The listing builds one solid part. Answer for the finished solid, in the listing's coordinates (mm). A direction names the side the tool comes from. Coordinates: 2 decimals unless noted, no trailing zeros. Order: outer loops, then holes, each group sorted by start corner. A loop starts at its lowest first (then second) coordinate and runs counter-clockwise, first axis right, second up. Notation, with made-up numbers: M 82.5,77 L 112.5,77 A23 ccw 112.5,91 Z; hole C 50,52.5 d3. An arc over 180 degrees is marked long. One line per item, written item: value. Start each with the question number.
Q1. The part is cut by section C-C on z = 12.6. Give the vertices of the cut face in (x, y), then the cut area to 3 significant figures.
Q2. Each of these flat-tipped pins is pushed along its axis until it touches: pin 1 Ø5 at (x, y) = (-13, 33) entering from -Z; pin 2 Ø12.5 at (y, z) = (13.5, 10) entering from -X; pin 3 Ø0.9 at (y, z) = (45.5, 35.5) entering from -X. Where does it stop, or does it pass through?
Q3. For faces 5 (the flat face through (-23.42, 54.41, 32.84)), 6 (the flat face through (1, 33, 0)), 7 (the flat face through (-29, 45, 35)), 8 (the flat face through (-19.5, 52, 29)), determine the directions among +Z, -Z, +X, -X, +Y, -Y from which every point of the face is accessible in a straight line to the end or side of a thin tool.
Q4. The part is cut by section B-B on y = 3.5. Give the vertices of the cut face in (x, z), then the cut area to 3 significant figures.
Q5. Determine the mould class of faces 1 (the flat face through (-28.65, 54.59, 33.86)), 2 (the flat face through (-9, 11, 12)), 3 (the cylindrical face through (-51.59, 52.94, 13.09)), 4 (the cylindrical face through (-57.526, 52.944, -2.419)) for opening direction X: pulls with the +X half, pulls with the -X half, needs draft (parallel to the pull), parting line crosses it, or undercut.
Q6. Straight lines are drawn through the part: line 1 along Y through (x, z) = (-44, 34); line 2 along Z through (x, y) = (3, 3); line 3 along Z through (x, y) = (-17, 18). For each, find the intervals that lie inside material, in ascending order. Write a range as [from, to].
Q7. The part is cut by section D-D on x = 4. Give the vertices of the cut face in (y, z).
Q8. The part is cut by section A-A on z = 28.1. Give the vertices of the cut face in (x, y).
```python
from build123d import *

# Parameters (mm, degrees)
BOSS_EXTRUDE1_DEPTH = 25.2
SKETCH2_R           = 1.6
BOSS_EXTRUDE2_DEPTH = 6
SKETCH3_W           = 19
SKETCH3_H           = 1
CUT_EXTRUDE1_DEPTH  = 38.2
CHAMFER2_SIZE       = 1.55
SKETCH4_R           = 11.1
CUT_EXTRUDE2_DEPTH  = 86.626222619
CHAMFER3_SIZE       = 1.55
CHAMFER4_SIZE       = 1
SKETCH5_R           = 1.6
CUT_EXTRUDE3_DEPTH  = 96.48869043
SKETCH6_W           = 20
SKETCH6_H           = 15
BOSS_EXTRUDE3_DEPTH = 3
SKETCH7_R           = 0.9
CUT_EXTRUDE4_DEPTH  = 95.097236941
CHAMFER7_SIZE       = 1.55
CHAMFER8_SIZE       = 1.55
SKETCH8_W           = 0.2
SKETCH8_H           = 55.2
CUT_EXTRUDE5_DEPTH  = 90.209024207
CHAMFER9_SIZE       = 1.6


with BuildPart() as part:
    # Sketch1 → Boss-Extrude1 (new body)
    with BuildSketch(Plane.XY):
        Polygon((0, 0), (0, 11), (-19, 11), (-19, 49.2), (8.8, 49.2), (8.8, 0), align=None)
    extrude(amount=BOSS_EXTRUDE1_DEPTH)

    # Sketch2 → Boss-Extrude2 (add)
    with BuildSketch(Plane(origin=(0, 49.2, 0), x_dir=(1, 0, 0), z_dir=(0, 1, 0))):
        Polygon((-61.5, 8.4), (-19.5, 8.4), (-19.5, 0), (8.8, 0), (8.8, -25.2), (-19.5, -25.2), (-19.5, -33.6), (-61.5, -33.6), align=None)
        with Locations(Location((-56, 2.9, 0), (0, 0, 180))):
            Circle(SKETCH2_R, mode=Mode.SUBTRACT)
        with Locations((-56, -28.1)):
            Circle(SKETCH2_R, mode=Mode.SUBTRACT)
        with Locations(Location((-25, -28.1, 0), (0, 0, 180))):
            Circle(SKETCH2_R, mode=Mode.SUBTRACT)
        with Locations((-25, 2.9)):
            Circle(SKETCH2_R, mode=Mode.SUBTRACT)
    extrude(amount=BOSS_EXTRUDE2_DEPTH)

    # Sketch3 → Cut-Extrude1 (cut)
    with BuildSketch(Plane.XZ.offset(-11)):
        with Locations((-9.5, 24.7)):
            Rectangle(SKETCH3_W, SKETCH3_H)
        with Locations((-9.5, 0.5)):
            Rectangle(SKETCH3_W, SKETCH3_H)
    extrude(amount=-CUT_EXTRUDE1_DEPTH, mode=Mode.SUBTRACT)

    # Chamfer2
    chamfer2_edges = [part.edges().sort_by_distance(p)[0] for p in [
        (-54.4, 49.2, -2.9),
        (-57.6, 49.2, 28.1),
        (-23.4, 49.2, 28.1),
        (-26.6, 49.2, -2.9),
    ]]
    chamfer(chamfer2_edges, length=CHAMFER2_SIZE)

    # Sketch4 → Cut-Extrude2 (cut, through all)
    with BuildSketch(Plane.XZ.offset(-49.2)):
        with Locations((-40.5, 12.6)):
            Circle(SKETCH4_R)
    extrude(amount=-CUT_EXTRUDE2_DEPTH, mode=Mode.SUBTRACT)

    # Chamfer3
    chamfer3_edges = [part.edges().sort_by_distance(p)[0] for p in [
        (-61.5, 55.2, 12.6),
        (-19.5, 52.2, 0),
        (-19.5, 52.2, -8.4),
        (-61.5, 49.2, 12.6),
        (-61.5, 52.2, -8.4),
        (-61.5, 52.2, 33.6),
        (-19.5, 52.2, 33.6),
        (-19.5, 52.2, 25.2),
        (-19, 30.1, 24.2),
        (-19, 30.1, 1),
        (-51.6, 49.2, 12.6),
    ]]
    chamfer(chamfer3_edges, length=CHAMFER3_SIZE)

    # Chamfer4
    chamfer4_edges = [part.edges().sort_by_distance(p)[0] for p in [
        (0, 30.1, 24.2),
        (0, 30.1, 1),
    ]]
    chamfer(chamfer4_edges, length=CHAMFER4_SIZE - 0.0001)  # a hair under: the kernel refuses the full size

    # Sketch5 → Cut-Extrude3 (cut, through all)
    with BuildSketch(Plane(origin=(8.8, 0, 0), x_dir=(0, 0, -1), z_dir=(1, 0, 0))):
        with Locations((-5.2, 3.5)):
            Circle(SKETCH5_R)
        with Locations(Location((-20, 3.5, 0), (0, 0, 180))):
            Circle(SKETCH5_R)
    extrude(amount=-CUT_EXTRUDE3_DEPTH, mode=Mode.SUBTRACT)

    # Sketch6 → Boss-Extrude3 (add)
    with BuildSketch(Plane.XY.offset(33.6)):
        with Locations((-39, 47.7)):
            Rectangle(SKETCH6_W, SKETCH6_H)
    extrude(amount=BOSS_EXTRUDE3_DEPTH)

    # Sketch7 → Cut-Extrude4 (cut, through all)
    with BuildSketch(Plane.XY.offset(36.6)):
        with Locations((-34, 45.2)):
            Circle(SKETCH7_R)
        with Locations((-44, 45.2)):
            Circle(SKETCH7_R)
    extrude(amount=-CUT_EXTRUDE4_DEPTH, mode=Mode.SUBTRACT)

    # Chamfer7
    chamfer7_edges = [part.edges().sort_by_distance(p)[0] for p in [
        (-29, 52.2, 33.6),
        (-25.025, 55.2, 33.6),
        (-29, 55.2, 35.1),
        (-49, 52.2, 33.6),
        (-49, 55.2, 35.1),
        (-54.475, 55.2, 33.6),
    ]]
    chamfer(chamfer7_edges, length=CHAMFER7_SIZE)

    # Chamfer8
    chamfer8_edges = [part.edges().sort_by_distance(p)[0] for p in [
        (-39, 55.2, 36.6),
    ]]
    chamfer(chamfer8_edges, length=CHAMFER8_SIZE)

    # Sketch8 → Cut-Extrude5 (cut, through all)
    with BuildSketch(Plane.XY.offset(25.2)):
        with Locations((8.7, 27.6)):
            Rectangle(SKETCH8_W, SKETCH8_H)
    extrude(amount=-CUT_EXTRUDE5_DEPTH, mode=Mode.SUBTRACT)

    # Chamfer9
    chamfer9_edges = [part.edges().sort_by_distance(p)[0] for p in [
        (8.6, 3.5, 6.8),
        (8.6, 3.5, 18.4),
    ]]
    chamfer(chamfer9_edges, length=CHAMFER9_SIZE)


solid = part.part
```
Output:
1. outline: M -61.5,50.75 L -59.95,49.2 L -53.15,49.2 L -51.6,50.75 L -51.6,55.2 L -59.95,55.2 L -61.5,53.65 Z; M -29.4,50.75 L -27.85,49.2 L -19,49.2 L -19,11 L 0,11 L 0,0 L 8.6,0 L 8.6,55.2 L -29.4,55.2 Z
1. area: 1,430 mm^2
2. pin 1: stops at z = 1
2. pin 2: stops at x = -19
2. pin 3: stops at x = -49
3. face 5: +Z, +X, +Y
3. face 6: -Z, +X, +Y, -Y
3. face 7: +Z, +X, -Y
3. face 8: +Z, +X, +Y, -Y
4. outline: M 0,0 L 8.6,0 L 8.6,2 L 7,3.6 L 0,3.6 Z; M 0,6.8 L 7,6.8 L 8.6,8.4 L 8.6,16.8 L 7,18.4 L 0,18.4 Z; M 0,21.6 L 7,21.6 L 8.6,23.2 L 8.6,25.2 L 0,25.2 Z
4. area: 157 mm^2
5. face 1: pulls with the +X half
5. face 2: needs draft
5. face 3: undercut
5. face 4: undercut
6. line 1: y = [40.2, 44.3], [46.1, 55.2]
6. line 2: z = [0, 3.68], [6.72, 18.48], [21.52, 25.2]
6. line 3: z = [1, 24.2]
7. outline: M 0,0 L 55.2,0 L 55.2,25.2 L 0,25.2 Z; hole C 3.5,5.2 d3.2; hole C 3.5,20 d3.2
8. outline: M -61.5,50.75 L -59.95,49.2 L -59.15,49.2 L -57.6,50.75 L -57.6,55.2 L -59.95,55.2 L -61.5,53.65 Z; M -54.4,50.75 L -52.85,49.2 L -28.15,49.2 L -26.6,50.75 L -26.6,55.2 L -54.4,55.2 Z; M -23.4,50.75 L -21.85,49.2 L -19.5,49.2 L -19.5,55.2 L -23.4,55.2 Z
